Design review of the part built by this model. Coordinates are the model's own, in mm. A direction names the side the tool comes from. Give positions to 0.01 mm unless a question says otherwise; leave off trailing zeros. Loops run counter-clockwise (first coordinate to the right, second up) from the corner with the lowest first, then second, coordinate; pieces in that order, holes last. Notation, with made-up numbers: (19, 47) - (66, 47) arc R24 cw to (66, 67) - close; hole circle Ø10 at (3.25, 0). An arc over 180 degrees is marked (long way). One line per item, written item: value. Start each with the question number.
```python
from build123d import *

# Parameters (mm, degrees)
SKETCH2_W                                     = 7.14375
SKETCH2_H                                     = 63.5
BOSS_EXTRUDE1_DEPTH                           = 114.3
CBORE_FOR_1_4_BUTTON_HEAD_CAP_SCREW1_AT_COUNT = 2
CBORE_FOR_1_4_BUTTON_HEAD_CAP_SCREW1_AT_PITCH = 82.55
CHAMFER1_SIZE                                 = 3.9624


with BuildPart() as part:
    # Sketch2 → Boss-Extrude1 (new body)
    with BuildSketch(Plane(origin=(0, 0, 0), x_dir=(0, 0, -1), z_dir=(1, 0, 0))):
        with Locations((3.571875, 31.75)):
            Rectangle(SKETCH2_W, SKETCH2_H)
    extrude(amount=-BOSS_EXTRUDE1_DEPTH)

    # Sketch3 → CBORE for 1/4 Button Head Cap Screw1 (revolve, cut)
    with BuildSketch(Plane(origin=(-98.425, 9.525, 0), x_dir=(0, -1, 0), z_dir=(1, 0, 0))):
        Polygon((0, 0), (0, 7.14375), (3.3782, 7.14375), (3.3782, 3.3528), (5.95376, 3.3528), (5.95376, 0.23749), (6.19125, 0), align=None)
    cbore_for_1_4_button_head_cap_screw1 = revolve(axis=Axis((-98.425, 9.525, 6.35), (0, 0, -1)), mode=Mode.SUBTRACT)

    # CBORE for 1/4 Button Head Cap Screw1 at: CBORE for 1/4 Button Head Cap Screw1 ×2
    with Locations(*[(i * CBORE_FOR_1_4_BUTTON_HEAD_CAP_SCREW1_AT_PITCH, 0, 0) for i in range(1, CBORE_FOR_1_4_BUTTON_HEAD_CAP_SCREW1_AT_COUNT)]):
        add(cbore_for_1_4_button_head_cap_screw1, mode=Mode.SUBTRACT)

    # Chamfer1
    chamfer1_edges = [part.edges().sort_by_distance(p)[0] for p in [
        (-57.15, 63.5, 0),
    ]]
    chamfer(chamfer1_edges, length=CHAMFER1_SIZE)


solid = part.part
```
(1) To check wall thickness, follow L1, parallel to X at y = 11, z = -4.5; L2, parallel to Z at x = -17, y = 5; L3, parallel to X at y = 4.5, z = -2.25. State the ranges of each line that lie inside material, in increasing order. Write a range as from..to.
(2) Take a section at A-A on x = -36.5. State the section outline as (y, z) points.
(3) Take a section at B-B on z = -1.5. State the section outline as (x, y) points (3 decimals), and give its area (3 significant figures).
(4) Take a section at C-C on y = 8. State how many separate pieces and enclosed holes the cut face has, and give its area (3 significant figures).
(5) Draft analysis for pull direction Y (two halves, no side actions). For faces 3 (the cylindrical face through (-13.595, 4.025, -1.773)), 4 (the flat face through (-114.3, 32, -4)), 5 (the flat face through (-13, 12, -3.353)), 6 (the flat face through (-56.35, 61.55, -2.01)), state which applies: pulls with the +Y half, pulls with the -Y half, needs draft (parallel to the pull), parting line crosses it, or undercut.
(6) For pin 1 Ø9.5 at (x, y) = (-98.425, 9.525) entering from +Z, flat-tipped, find the tip position at first contact; note if it passes through.
(7) Machinability: for faces 1 (the flat face through (-95.9, 12.1, -3.353)), 2 (the cylindrical face through (-95.428, 7.966, -5.222)), which of the approach directions +Z, -Z, +X, -X, +Y, -Y give a long, thin tool a straight path to every point of the face, cutting with its end or side? Answer none if there is none.
Here are the results:
1. L1: -114.3..-101.46, -95.39..-18.91, -12.84..0
1. L2: -7.14..-3.35
1. L3: -114.3..-101.62, -95.23..-19.07, -12.68..0
2. outline: (0, -7.14) - (63.5, -7.14) - (63.5, -3.96) - (59.54, 0) - (0, 0) - close
3. outline: (-114.3, 0) - (0, 0) - (0, 61.038) - (-114.3, 61.038) - close; hole circle Ø11.908 at (-98.425, 9.525); hole circle Ø11.908 at (-15.875, 9.525)
3. area: 6,750 mm²
4. separate pieces: 3
4. enclosed holes: 0
4. area: 694 mm²
5. face 3: undercut
5. face 4: needs draft
5. face 5: undercut
5. face 6: pulls with the +Y half
6. pin 1: z = -3.35
7. face 1: +Z
7. face 2: +Z, -Z
